Part model, mm, in its own coordinate system. Coordinates: 2 decimals unless noted, no trailing zeros. Write each loop counter-clockwise with the first axis right and the second up, starting at its lowest first coordinate (ties: lowest second). Pieces come first, ordered by that corner, then holes. Notation, with made-up numbers: (72, 10) - (83, 10) arc R18 ccw to (83, 40) - close; hole circle Ø1 at (39.5, 43). An arc over 180 degrees is marked (long way). Use a Markdown table: item, result.
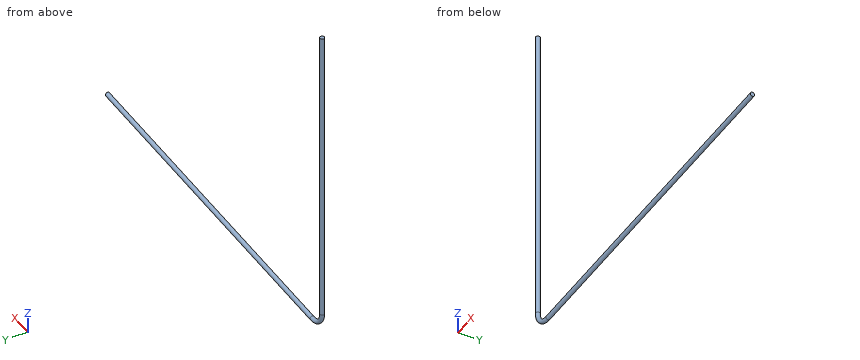
Autodesk Inventor part; units mm, degrees
ref_plane "Work Plane1" through (76.2, 0, 0) normal (1, 0, 0) x (0, 1, 0)
ref_plane "XZ Plane" through (0, 0, 0) normal (0, 1, 0) x (-1, 0, 0)
ref_plane "XY Plane" through (0, 0, 0) normal (0, 0, 1) x (1, 0, 0)
sketch "Sketch2" plane through (0, 0, 0) normal (0, 0, 1) x (1, 0, 0)
  circle A0 centre (0, 0) radius 9.525
  dimension "d3" = 19.05
extrude "Extrusion2" add sketch "Sketch2" against normal blind 1365.25
ref_plane "Work Plane1" through (76.2, 0, 0) normal (1, 0, 0) x (0, 1, 0)
sketch "Sketch9" plane through (76.2, 0, 0) normal (1, 0, 0) x (0, 1, 0)
  line L0 (-9.525, -1365.25) -> (9.525, -1365.25)
  circle A0 centre (0, -1441.45) radius 9.525
  line L1 (0, -1365.25) -> (0, -1441.45) construction
  point P0 (0, 0)
  dimension "d17" = 19.05
  dimension "d18" = 76.2
extrude "Extrusion4" add sketch "Sketch9" along normal blind 1543.05
sketch "Sketch11" plane through (0, 0, -1365.25) normal (0, 0, -1) x (-1, 0, 0)
  circle A0 centre (0, 0) radius 9.525
sketch "Sketch12" plane through (0, 0, 0) normal (0, 1, 0) x (-1, 0, 0)
  line L0 (-76.2, -1450.975) -> (-76.2, -1431.925)
  line L1 (-9.525, -1365.25) -> (9.525, -1365.25)
  arc A0 (-76.2, -1441.45) -> (0, -1365.25) centre (-76.2, -1365.25) ccw
  point P0 (0, 0)
  dimension "d21" = 76.2
sweep "Sweep2" add profiles "Sketch11" path "Sketch12" path curves A0
equation "\"d3\" = tubeD"
equation "\"d17\" = tubeD"
equation "\"d18\" = tubeTurnR"
equation "\"d21\" = tubeTurnR"
equation "\"d4\" = tubeTurnR"
equation "\"wallThick\" = 44.45"
equation "\"roomWidth\" = 3048"
equation "\"roomDepth\" = 3657.6"
equation "\"roomHeight\" = 2438.4"
equation "\"doorWidth\" = 895.35"
equation "\"doorHeight\" = 2108.2"
equation "\"doorX\" = 774.7"
equation "\"doorY\" = 88.9"
equation "\"doorLip\" = 76.2"
equation "\"doorThick\" = 57.15"
equation "\"tubeTurnR\" = 76.2"
equation "\"tubeD\" = 19.05"
properties part number "left_tube_0"
Item 1: Band-saw the part on B-B, the plane x = 1016.5. Give the cut face in (y, z) (3 decimals).
From the geometry:
| item | result |
|---|---|
| outline | circle Ø19.05 at (0, -1441.45) |
Item 2: Drill centre lines: probe 1 along X at (y, z) = (2.25, -65); probe 2 along X at (y, z) = (1.5, -392.5); probe 3 along Z at (x, y) = (1061, -1). Where is each one in solid material? Low to high.
From the geometry:
| item | result |
|---|---|
| probe 1 | -9.26 to 9.26 |
| probe 2 | -9.41 to 9.41 |
| probe 3 | -1450.92 to -1431.98 |
Item 3: Band-saw the part on C-C, the plane z = -774. Give the cut face in (x, y) (3 decimals).
From the geometry:
| item | result |
|---|---|
| outline | circle Ø19.05 at (0, 0) |
Item 4: Band-saw the part on A-A, the plane y = 4.75. Give the cut face in (x, z), then the cut area to 3 significant figures.
From the geometry:
| item | result |
|---|---|
| outline | (-8.26, -1365.25) arc R84.46 ccw to (76.2, -1449.71) - (1619.25, -1449.71) - (1619.25, -1433.19) - (76.2, -1433.19) arc R67.94 cw to (8.26, -1365.25) - (8.26, 0) - (-8.26, 0) - close |
| area | 50,000 mm^2 |
Item 5: Drop flat-ended pins along their axis: P1, Ø3, axis at x = 784, y = 5.5, coming from the +Z side; P2, Ø10, axis at y = 3, z = -780, coming from the +X side (3 decimals); P3, Ø1, axis at x = 1270, y = -2.5, coming from the -Z side. Give the stop position or say it passes through.
From the geometry:
| item | result |
|---|---|
| P1 | z = -1432.81 |
| P2 | x = 9.525 |
| P3 | z = -1450.76 |
